The figure shows three views and two pictorial views of one solid part (mm, origin at its lowest corner). Answer the questions. Give positions to 0.01 mm unless a question says otherwise; leave off trailing zeros. Order: outer loops, then holes, each group sorted by start corner. A loop starts at its lowest first (then second) coordinate and runs counter-clockwise, first axis right, second up. Notation, with made-up numbers: M 50,-33.5 L 106,-33.5 A8 cw 106,-19.5 Z; hole C 22,32.25 d7. An arc over 180 degrees is marked long. One line per item, written item: value.
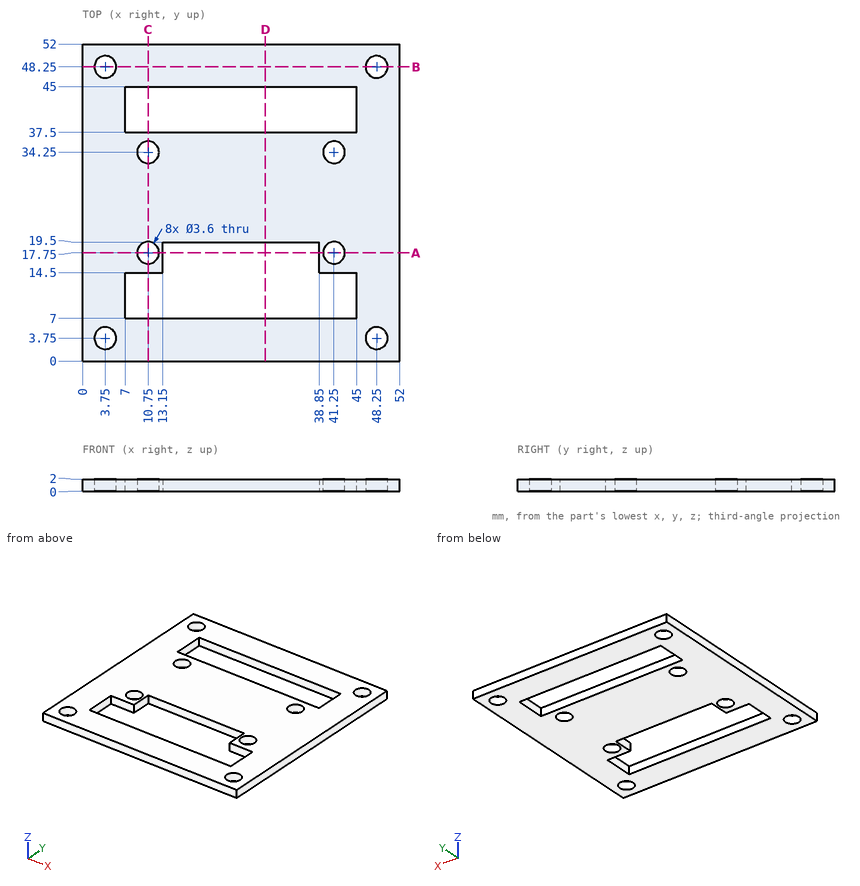
1) Find section A-A, the plane y = 17.75. Write down the section's boundary in (x, z), plus the area to 3 significant figures.
Reported:
outline: M 0,0 L 8.95,0 L 8.95,2 L 0,2 Z; M 12.55,0 L 13.15,0 L 13.15,2 L 12.55,2 Z; M 38.85,0 L 39.45,0 L 39.45,2 L 38.85,2 Z; M 43.05,0 L 52,0 L 52,2 L 43.05,2 Z
area: 38.2 mm^2
2) Consider probe 1 along Y at (x, z) = (48.25, 0.75); probe 2 along Y at (x, z) = (10.75, 1.55); probe 3 along Y at (x, z) = (26, 1.85). Determine where each line is inside the solid, lowest interval first.
Reported:
probe 1: y = 0 to 1.95, 5.55 to 46.45, 50.05 to 52
probe 2: y = 0 to 7, 14.5 to 15.95, 19.55 to 32.45, 36.05 to 37.5, 45 to 52
probe 3: y = 0 to 7, 19.5 to 37.5, 45 to 52
3) Find section C-C, the plane x = 10.75. Write down the section's boundary in (y, z).
Reported:
outline: M 0,0 L 7,0 L 7,2 L 0,2 Z; M 14.5,0 L 15.95,0 L 15.95,2 L 14.5,2 Z; M 19.55,0 L 32.45,0 L 32.45,2 L 19.55,2 Z; M 36.05,0 L 37.5,0 L 37.5,2 L 36.05,2 Z; M 45,0 L 52,0 L 52,2 L 45,2 Z
4) Each of these flat-tipped pins is pushed along its axis until it touches: pin 1 Ø5 at (x, y) = (37, 42) entering from +Z; pin 2 Ø0.6 at (x, z) = (33.5, 1) entering from -Y. Where does it stop, or does it pass through?
Reported:
pin 1: passes through
pin 2: stops at y = 0
5) Find section D-D, the plane x = 30. Write down the section's boundary in (y, z).
Reported:
outline: M 0,0 L 7,0 L 7,2 L 0,2 Z; M 19.5,0 L 37.5,0 L 37.5,2 L 19.5,2 Z; M 45,0 L 52,0 L 52,2 L 45,2 Z
6) Find section B-B, the plane y = 48.25. Write down the section's boundary in (x, z), plus the area to 3 significant figures.
Reported:
outline: M 0,0 L 1.95,0 L 1.95,2 L 0,2 Z; M 5.55,0 L 46.45,0 L 46.45,2 L 5.55,2 Z; M 50.05,0 L 52,0 L 52,2 L 50.05,2 Z
area: 89.6 mm^2
